```python
from build123d import *

# Parameters (mm, degrees)
SKETCH1_R          = 55.5
BASE_FLANGE1_DEPTH = 20


# Sheet-metal steps are written as plain solids
with BuildPart() as part:
    # Sketch1 → Base-Flange1 (new body)
    with BuildSketch(Plane(origin=(0, 0, 0), x_dir=(0, 0, -1), z_dir=(1, 0, 0))):
        with BuildLine():
            Line((0, -41), (0, -12.5))
            ThreePointArc((0, -12.5), (3.661165235, -3.661165235), (12.5, 0))
            Line((12.5, 0), (402, 0))
            Line((402, 0), (404.831276436, 219.451346471))
            ThreePointArc((404.831276436, 219.451346471), (353.919996754, 296.731364001), (263.269941068, 278.110759489))
            ThreePointArc((263.269941068, 278.110759489), (113.107275555, 187.171901633), (-62.321618696, 180.583651161))
            ThreePointArc((-62.321618696, 180.583651161), (-154.024103093, 136.42364838), (-133.058215758, 36.825038658))
            Line((-133.058215758, 36.825038658), (-45.972209781, -36.315142143))
            ThreePointArc((-45.972209781, -36.315142143), (-39.95421417, -39.792323471), (-33.109612021, -41))
            Line((-33.109612021, -41), (0, -41))
        make_face()
        with Locations((-80, 100)):
            Circle(SKETCH1_R, mode=Mode.SUBTRACT)
        with Locations((322.338141708, 220.515641005)):
            Circle(SKETCH1_R, mode=Mode.SUBTRACT)
    extrude(amount=-BASE_FLANGE1_DEPTH)


solid = part.part
```
The model under review builds one solid part; all positions refer to its coordinate system, in mm. Give positions to 0.01 mm unless a question says otherwise; leave off trailing zeros. Order: outer loops, then holes, each group sorted by start corner. A loop starts at its lowest first (then second) coordinate and runs counter-clockwise, first axis right, second up. Notation, with made-up numbers: (-7, 31.25) - (13, 31.25) arc R31 ccw to (13, 65.25) - close; hole circle Ø8 at (35.25, 34). An arc over 180 degrees is marked (long way). Use CSV: the item, a comma, the result in double quotes. Start each with the question number.
Q1. We need section A-A, the plane y = 100. Write out the cut boundary in (x, z), and give its area (3 significant figures).
Q2. We need section C-C, the plane x = -9. Write out the cut boundary in (y, z).
Q3. We need section B-B, the plane z = 97. Write out the cut boundary in (x, y).
Q4. The part is to be moulded in two halves that separate along Z. For faces 1 (the flat face through (-10, -27, 0)), 2 (the flat face through (-10, 0, -205)), 3 (the cylindrical face through (-9.86, 146.798, 50.164)), say which applies: +Z half, -Z half, draft (parallel to the pull), parting line (faces both ways), or undercut.
Q5. We need section D-D, the plane z = -57.5. Write out the cut boundary in (x, y).
Q6. To check wall thickness, follow line 1 along Y through (x, z) = (-6, 80); line 2 along Z through (x, y) = (-13.25, 225); line 3 along Z through (x, y) = (-9, 51). State the ranges of each line that lie inside material, in increasing order. Write a range as [from, to].
Q7. Clearance check with flat-ended pins moving along their axes: pin 1 Ø1.5 at (x, y) = (-13, 174) entering from +Z; pin 2 Ø3 at (x, y) = (-11.5, 42.5) entering from -Z; pin 3 Ø4 at (x, z) = (-18, 90.5) entering from -Y. State where each tip first meets the part, or that it passes through.
Outcome:
1,outline,"(-20, -403.29) - (0, -403.29) - (0, 24.5) - (-20, 24.5) - close; (-20, 135.5) - (0, 135.5) - (0, 162.5) - (-20, 162.5) - close"
1,area,"9,100 mm^2"
2,outline,"(-41, 0) - (-12.5, 0) arc R12.5 cw to (0, -12.5) - (0, -402) - (219.45, -404.83) arc R82.5 ccw to (278.11, -263.27) arc R350 cw to (180.58, 62.32) arc R82.5 ccw to (36.83, 133.06) - (-36.32, 45.97) arc R20 ccw to (-41, 33.11) - close; hole circle Ø111 at (100, 80); hole circle Ø111 at (220.52, -322.34)"
3,outline,"(-20, 6.54) - (0, 6.54) - (0, 47.17) - (-20, 47.17) - close; (-20, 152.83) - (0, 152.83) - (0, 180.73) - (-20, 180.73) - close"
4,face 1,"-Z half"
4,face 2,"draft"
4,face 3,"undercut"
5,outline,"(-20, 0) - (0, 0) - (0, 175.34) - (-20, 175.34) - close"
6,line 1,"y = [-7.74, 44.5], [155.5, 182.5]"
6,line 2,"z = [-404.72, -377.66], [-267.02, -197.13]"
6,line 3,"z = [-402.66, 53.94], [106.06, 146.37]"
7,pin 1,"stops at z = 117.96"
7,pin 2,"stops at z = -402.57"
7,pin 3,"stops at y = -0.6"
